For this review, take the finished solid that the model builds, in its own axes (mm). A direction names the side the tool comes from. Round coordinates to 2 decimals unless told otherwise and drop trailing zeros. Write each loop counter-clockwise with the first axis right and the second up, starting at its lowest first coordinate (ties: lowest second). Pieces come first, ordered by that corner, then holes. Notation, with made-up numbers: M 88,5 L 103,5 A25 ccw 103,38 Z; hole C 18.25,-2.5 d5. An arc over 180 degrees is marked long. Answer in a Markdown table with one row per item.
```python
from build123d import *

# Parameters (mm, degrees)
BOSS_EXTRUDE1_DEPTH = 4.5593
CAVITY1_START       = -26.67
CAVITY1_OUTLINE_W   = 12.49172
CAVITY1_OUTLINE_H   = 4.5593
CAVITY1_OUTLINE_W_2 = 7.93242
CAVITY1_DEPTH       = 4.5593


# Read off the part's stored shape, not the designer's step: Cavity1
with BuildPart() as part:
    # Sketch1 → Boss-Extrude1 (new body)
    with BuildSketch(Plane.XY):
        Polygon((31.2293, 0), (31.2293, 3.27152), (-26.67, 3.27152), (-26.67, 0), (-31.2293, 0), (-31.2293, -8.89), (-26.67, -8.89), (-26.67, -17.78), (-31.2293, -17.78), (-31.2293, -26.67), (26.67, -26.67), (26.67, -17.78), (31.2293, -17.78), (31.2293, -8.89), (26.67, -8.89), (26.67, 0), align=None)
    extrude(amount=BOSS_EXTRUDE1_DEPTH)

    # Cavity1 outline → Cavity1 (cut)
    with BuildSketch(Plane(origin=(0, 0, 0), x_dir=(1, 0, 0), z_dir=(0, 1, 0)).offset(CAVITY1_START)):
        with Locations((-24.98344, -2.27965)):
            Rectangle(CAVITY1_OUTLINE_W, CAVITY1_OUTLINE_H)
        with Locations((0, -2.27965)):
            Rectangle(CAVITY1_OUTLINE_W, CAVITY1_OUTLINE_H)
        with Locations((22.70379, -2.27965)):
            Rectangle(CAVITY1_OUTLINE_W_2, CAVITY1_OUTLINE_H)
    extrude(amount=CAVITY1_DEPTH, mode=Mode.SUBTRACT)


solid = part.part
```
Q1. Take a section at A-A (z = 3.85). State the section outline as (x, y) points, then the cut area to 3 significant figures.
Found:
| item | result |
|---|---|
| outline | M -31.23,-22.11 L -18.74,-22.11 L -18.74,-26.67 L -6.25,-26.67 L -6.25,-22.11 L 6.25,-22.11 L 6.25,-26.67 L 18.74,-26.67 L 18.74,-22.11 L 26.67,-22.11 L 26.67,-17.78 L 31.23,-17.78 L 31.23,-8.89 L 26.67,-8.89 L 26.67,0 L 31.23,0 L 31.23,3.27 L -26.67,3.27 L -26.67,0 L -31.23,0 L -31.23,-8.89 L -26.67,-8.89 L -26.67,-17.78 L -31.23,-17.78 Z |
| area | 1,580 mm² |
Q2. Machinability: for faces 4 (the face through (6.246, -24, 2)), 5 (the face through (18.738, -24, 2)), 6 (the face through (-25, -22.111, 2)), which of the approach directions +Z, -Z, +X, -X, +Y, -Y give a long, thin tool a straight path to every point of the face, cutting with its end or side? Answer none if there is none.
Found:
| item | result |
|---|---|
| face 4 | +Z, -Z, -Y |
| face 5 | +Z, -Z, +X, -Y |
| face 6 | +Z, -Z, -X, -Y |
Q3. For probe 1 along X at (y, z) = (-22.25, 2.2); probe 2 along X at (y, z) = (-3.25, 3); probe 3 along X at (y, z) = (2, 2.05), list the stretches that pass through material, from the lowest coordinate up.
Found:
| item | result |
|---|---|
| probe 1 | -18.74 to -6.25, 6.25 to 18.74 |
| probe 2 | -31.23 to 26.67 |
| probe 3 | -26.67 to 31.23 |
Q4. Take a section at B-B (y = -3). State the section outline as (x, z) points.
Found:
| item | result |
|---|---|
| outline | M -31.23,0 L 26.67,0 L 26.67,4.56 L -31.23,4.56 Z |
Q5. Insertion check: P1, Ø1.4, axis at x = -29, z = 3, coming from the -Y side; P2, Ø2.5, axis at y = 2, z = 2.5, coming from the -X side; P3, Ø2.5, axis at y = -4.5, z = 1.5, coming from the +X side. Each pin has a flat end and moves straight along its axis. Give the tip position at first contact, or say it passes through.
Found:
| item | result |
|---|---|
| P1 | y = -22.11 |
| P2 | x = -26.67 |
| P3 | x = 26.67 |
Q6. Mouldability with a two-part tool opening along Y and no side actions: class faces 1 (the face through (0, -11, 0)), 2 (the face through (29, 0, 2)), 3 (the face through (-29, 0, 2)) as +Y half, -Y half, draft (parallel to the pull), parting line (faces both ways), or undercut.
Found:
| item | result |
|---|---|
| face 1 | draft |
| face 2 | undercut |
| face 3 | +Y half |
Q7. Take a section at C-C (x = 4.5). State the section outline as (y, z) points.
Found:
| item | result |
|---|---|
| outline | M -22.11,0 L 3.27,0 L 3.27,4.56 L -22.11,4.56 Z |
